```python
from build123d import *

# Parameters (mm, degrees)
F0_R          = 15.625
F0_R_2        = 5.715
F1_DEPTH      = 20
F2_R          = 5.715
F2_R_2        = 4.70576
F3_DEPTH      = 2.01848
F3_DEPTH_BACK = 22.01848
F4_R          = 20.5
F4_R_2        = 5.715
F5_DEPTH      = 2.01848
F6_R          = 20.5
F6_R_2        = 5.715
F7_DEPTH      = 2.01848


with BuildPart() as f1:
    # F0 (on Top) → F1 (new body)
    with BuildSketch(Plane.XY):
        Circle(F0_R)
        Circle(F0_R_2, mode=Mode.SUBTRACT)
    extrude(amount=F1_DEPTH)

    # F2 (on face) → F3 (join, two sides)
    with BuildSketch(Plane.XY.offset(20)) as f3_sk:
        Circle(F2_R)
        Circle(F2_R_2, mode=Mode.SUBTRACT)
    extrude(amount=F3_DEPTH)
    extrude(f3_sk.sketch, amount=-F3_DEPTH_BACK)

    # F4 (on face) → F5 (join)
    with BuildSketch(Plane.XY.offset(20)):
        Circle(F4_R)
        Circle(F4_R_2, mode=Mode.SUBTRACT)
    extrude(amount=F5_DEPTH)

    # F6 (on face) → F7 (join)
    with BuildSketch(Plane(origin=(0, 0, 0), x_dir=(1, 0, 0), z_dir=(0, 0, -1))):
        Circle(F6_R)
        Circle(F6_R_2, mode=Mode.SUBTRACT)
    extrude(amount=F7_DEPTH)


solid = f1.part
```
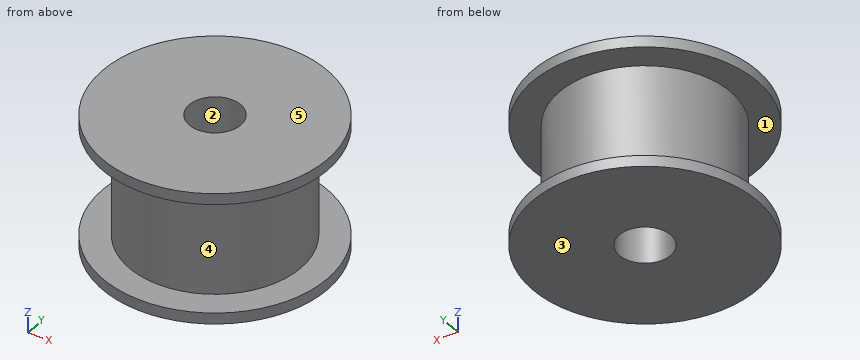
Source: CAD feature listing. Evaluate the final solid. Frame: model axes, mm. Face numbers are marked on the shaded views. A direction names the side the tool comes from. Give positions to 0.01 mm unless a question says otherwise; leave off trailing zeros. Write each loop counter-clockwise with the first axis right and the second up, starting at its lowest first coordinate (ties: lowest second). Pieces come first, ordered by that corner, then holes.
1. Section query D-D (x = 12.5). Return the cut outline in (y, z) (3 decimals).
2. Section query A-A (x = 0). Return the cut outline in (y, z) (3 decimals), then the cut area to 3 significant figures.
3. Material intervals for line 1 along Z through (x, y) = (8, -17); line 2 along Y through (x, z) = (0, 12) (3 decimals); line 3 along X through (y, z) = (-2, 15), sorted ascending.
4. Section query C-C (z = 3). Return the cut outline in (x, y) (3 decimals), then the cut area to 3 significant figures.
5. First-contact query: pin 1 (10 mm diameter, centred on x = -15.5, z = 19.5, fed in from +Y); pin 2 (1.5 mm diameter, centred on y = -0.5, z = 18.5, fed in from -X) (3 decimals); pin 3 (2 mm diameter, centred on y = 5, z = 13, fed in from -X). Flat tips, straight axial feed; report the tip coordinate or a pass-through.
6. Access query for the marked faces 1 and 2. Directions: +Z, -Z, +X, -X, +Y, -Y. A direction counts if a zero-diameter tool reaches every point of the face in a straight line with its end or side. Return the directions, or none.
7. Pull-direction query (Z, two-part tool) for the marked faces 3, 4 and 5; classes: +Z half, -Z half, draft (parallel to the pull), parting line (faces both ways), or undercut.
Output values:
1. outline: (-16.248, -2.018) - (16.248, -2.018) - (16.248, 0) - (9.375, 0) - (9.375, 20) - (16.248, 20) - (16.248, 22.018) - (-16.248, 22.018) - (-16.248, 20) - (-9.375, 20) - (-9.375, 0) - (-16.248, 0) - close
2. outline: (-20.5, -2.018) - (-4.706, -2.018) - (-4.706, 22.018) - (-20.5, 22.018) - (-20.5, 20) - (-15.625, 20) - (-15.625, 0) - (-20.5, 0) - close; (4.706, -2.018) - (20.5, -2.018) - (20.5, 0) - (15.625, 0) - (15.625, 20) - (20.5, 20) - (20.5, 22.018) - (4.706, 22.018) - close
2. area: 564 mm2
3. line 1: z = -2.02 to 0, 20 to 22.02
3. line 2: y = -15.625 to -4.706, 4.706 to 15.625
3. line 3: x = -15.5 to -4.26, 4.26 to 15.5
4. outline: circle Ø31.25 at (0, 0); hole circle Ø9.412 at (0, 0)
4. area: 697 mm2
5. pin 1: stops at y = 17.59
5. pin 2: stops at x = -15.625
5. pin 3: stops at x = -15.1
6. face 1: none
6. face 2: +Z, -Z
7. face 3: -Z half
7. face 4: undercut
7. face 5: +Z half
